For this review, take the finished solid that the model builds, in its own axes (mm). A direction names the side the tool comes from. Round coordinates to 2 decimals unless told otherwise and drop trailing zeros. Write each loop counter-clockwise with the first axis right and the second up, starting at its lowest first coordinate (ties: lowest second). Pieces come first, ordered by that corner, then holes. Notation, with made-up numbers: (7, 88) - (18, 88) arc R13 cw to (18, 93) - close; hole circle Ø9 at (51.25, 32.25). An arc over 180 degrees is marked (long way). One line per item, written item: value. Start each with the question number.
Q1. Add section A-A on z = 0. Write out the cut boundary in (x, y), and give its area (3 significant figures).
Q2. Mouldability with a two-part tool opening along Z and no side actions: class faces 4 (the face through (9.86, 39.1, -13.26)), 5 (the face through (11.613, -42.338, 10.114)), 6 (the face through (9.86, -7.06, 40.42)) as +Z half, -Z half, draft (parallel to the pull), parting line (faces both ways), or undercut.
Q3. Clearance check with flat-ended pins moving along their axes: pin 1 Ø16 at (y, z) = (-34.33, 36.35) entering from +X; pin 2 Ø3 at (x, y) = (16.5, -22.5) entering from +Z; pin 3 Ø8 at (x, y) = (5, -18) entering from +Z; pin 4 Ø4 at (x, y) = (9, -34) entering from -Z. State where each tip first meets the part, or that it passes through.
Q4. Add section C-C on x = 9.75. Write out the cut boundary in (y, z), and give its area (3 significant figures).
Q5. Add section D-D on z = -22.5. Write out the cut boundary in (x, y), and give its area (3 significant figures).
Q6. Add section B-B on y = 54. Write out the cut boundary in (x, z).
Q7. For probe 1 along Z at (x, y) = (17, 48); probe 2 along Z at (x, y) = (11.5, -22.5); probe 3 along Y at (x, z) = (2.5, 20), list the stretches that pass through material, from the lowest coordinate up.
Q8. Tool access review of faces 1 (the face through (10, -22, 28)), 2 (the face through (9.86, 13.136, -38.386)), 3 (the face through (9.9, 27.7, 30.3)): name each direction out of +Z, -Z, +X, -X, +Y, -Y from which nothing blocks a thin tool from reaching the whole face with its end or side.
```python
from build123d import *

# Parameters (mm, degrees)
F0_R     = 10
F1_DEPTH = 20
F2_R     = 3
F3_DEPTH = 2.5
F4_W     = 12
F4_H     = 12
F5_DEPTH = 30


with BuildPart() as f1:
    # F0 (on Right) → F1 (new body)
    with BuildSketch(Plane.YZ):
        with BuildLine():
            Line((7.481455, 29.052157), (-22.012425, 52.10852))
            ThreePointArc((-22.012425, 52.10852), (-47.949661, 50.997752), (-50.938718, 25.20939))
            Line((-50.938718, 25.20939), (-29.07978, -7.373356))
            ThreePointArc((-29.07978, -7.373356), (-21.17372, 21.252614), (7.481455, 29.052157))
        make_face()
        with Locations((-34.330039, 36.351732)):
            Circle(F0_R, mode=Mode.SUBTRACT)
        with BuildLine():
            Line((47.414482, 31.516835), (7.481455, 29.052157))
            ThreePointArc((7.481455, 29.052157), (23.711217, 18.378742), (30, 0))
            ThreePointArc((30, 0), (28.223022, -10.17158), (23.102597, -19.138182))
            Line((23.102597, -19.138182), (55.544301, -7.218058))
            ThreePointArc((55.544301, -7.218058), (68.220071, 15.662983), (47.414482, 31.516835))
        make_face()
        with Locations((48.646543, 11.55482)):
            Circle(F0_R, mode=Mode.SUBTRACT)
        with BuildLine():
            ThreePointArc((23.102597, -19.138182), (-6.598065, -29.265432), (-29.07978, -7.373356))
            Line((-29.07978, -7.373356), (-33.994642, -44.332917))
            Line((-33.994642, -44.332917), (-34.244702, -46.213358))
            ThreePointArc((-34.244702, -46.213358), (-19.868232, -67.120566), (3.443665, -57.103095))
            Line((3.443665, -57.103095), (23.102597, -19.138182))
        make_face()
        with Locations((-14.316504, -47.906552)):
            Circle(F0_R, mode=Mode.SUBTRACT)
        with BuildLine():
            ThreePointArc((30, 0), (23.711217, 18.378742), (7.481455, 29.052157))
            ThreePointArc((7.481455, 29.052157), (-21.17372, 21.252614), (-29.07978, -7.373356))
            ThreePointArc((-29.07978, -7.373356), (-6.598065, -29.265432), (23.102597, -19.138182))
            ThreePointArc((23.102597, -19.138182), (28.223022, -10.17158), (30, 0))
        make_face()
        Circle(F0_R, mode=Mode.SUBTRACT)
    extrude(amount=F1_DEPTH)

    # F2 (on face) → F3 (join, symmetric)
    with BuildSketch(Plane(origin=(0, -23.46529, -15.742268), x_dir=(1, 0, 0), z_dir=(0, -0.830434, -0.557117))):
        with Locations((10, 29.456303)):
            Circle(F2_R)
    extrude(amount=F3_DEPTH, both=True)

    # F4 (on face) → F5 (cut)
    with BuildSketch(Plane.YZ.offset(20)):
        with Locations((-22, 22)):
            Rectangle(F4_W, F4_H)
    extrude(amount=-F5_DEPTH, mode=Mode.SUBTRACT)


solid = f1.part
```
Result set:
1. outline: (0, -34.03) - (20, -34.03) - (20, -10) - (0, -10) - close; (0, 10) - (20, 10) - (20, 64.97) - (0, 64.97) - close
1. area: 1,580 mm^2
2. face 4: -Z half
2. face 5: undercut
2. face 6: +Z half
3. pin 1: passes through
3. pin 2: stops at z = 53.48
3. pin 3: stops at z = 52.1
3. pin 4: stops at z = -57.25
4. outline: (-50.94, 25.21) - (-41.54, 11.2) - (-43.62, 9.81) - (-40.29, 4.84) - (-38.21, 6.24) - (-29.08, -7.37) - (-34.24, -46.21) arc R20 ccw to (3.44, -57.1) - (23.1, -19.14) - (55.54, -7.22) arc R20 ccw to (47.41, 31.52) - (7.48, 29.05) - (-22.01, 52.11) arc R20 ccw to start; hole circle Ø20 at (-34.33, 36.35); hole (-28, 16) - (-16, 16) - (-16, 28) - (-28, 28) - close; hole circle Ø20 at (-14.32, -47.91); hole circle Ø20 at (0, 0); hole circle Ø20 at (48.65, 11.55)
4. area: 6,520 mm^2
5. outline: (0, -31.09) - (20, -31.09) - (20, 21.36) - (0, 21.36) - close
5. area: 1,050 mm^2
6. outline: (0, -7.79) - (20, -7.79) - (20, 3.11) - (0, 3.11) - close; (0, 20) - (20, 20) - (20, 30.83) - (0, 30.83) - close
7. probe 1: z = -9.99 to 1.58, 21.53 to 31.54
7. probe 2: z = -66.16 to -53.65, -42.16 to 16, 28 to 52.48
7. probe 3: y = -47.44 to -28, -16 to 43.29, 54 to 66.78
8. face 1: +X, -X
8. face 2: -Z, +X, -X, +Y
8. face 3: +Z, +X, -X
